Part model, mm, in its own coordinate system. A direction names the side the tool comes from. Coordinates: 2 decimals unless noted, no trailing zeros. Loops run counter-clockwise (first coordinate to the right, second up) from the corner with the lowest first, then second, coordinate; pieces in that order, holes last. Notation, with made-up numbers: M -19,-27.75 L 39,-27.75 A6 ccw 39,-17.75 Z; hole C 8.5,84.25 d5. An arc over 180 degrees is marked long. Use a Markdown table: item, result. Add a question column.
1) Tool access for faces 1 (the cylindrical face through (-1.46, 3.49, 6.59)), 2 (the flat face through (-2, 3, -6)): list every direction of +Z, -Z, +X, -X, +Y, -Y with a clear straight run to the whole face (end or side of a thin tool).
2) Pull direction Z, two halves, no side cores. Call faces 3 (the cylindrical face through (0, 2, 2)), 4 (the flat face through (-1, 4, -2)), 5 (the cylindrical face through (-6, 2, 0)): released by +Z, released by -Z, zero draft, split by the parting line, or undercut.
3) Band-saw the part on A-A (z = 0). List the corners of the cut face in (x, y).
4) Band-saw the part on C-C (y = 1.7). List the corners of the cut face in (x, z), plus the area to 3 significant figures.
5) Wall check: probe 1 along Z at (x, y) = (0, 1.35); probe 2 along Y at (x, z) = (-0.75, 6). Give the ranges that are in metal, low to high. Write a range as from..to.
6) Band-saw the part on B-B (x = 0). List the corners of the cut face in (y, z), plus the area to 3 significant figures.
7) Pin check, flat tips, straight feed: pin 1 Ø2 at (x, y) = (4, 2.5) entering from -Z; pin 2 Ø2 at (y, z) = (1.5, -5) entering from -X. Stop position of each tip, or through.
from build123d import *

# Parameters (mm, degrees)
CHAMFER_1_SIZE = 0.1


with BuildPart() as part:
    # 草图1 → 旋转1 (revolve)
    with BuildSketch(Plane.XY):
        Polygon((2, 0), (2, 4), (6.75, 4), (6.75, 3), (6, 3), (6, 0), align=None)
    revolve(axis=Axis((0, 0, 0), (0, 1, 0)))

    # 倒角1
    chamfer_1_edges = [part.edges().sort_by_distance(p)[0] for p in [
        (-6, 0, 0),
        (-6.75, 3, 0),
        (-6.75, 4, 0),
    ]]
    chamfer(chamfer_1_edges, length=CHAMFER_1_SIZE)


solid = part.part
Entries:
| question | item | result |
|---|---|---|
| 1 | face 1 | +Y, -Y |
| 1 | face 2 | -Y |
| 2 | face 3 | undercut |
| 2 | face 4 | zero draft |
| 2 | face 5 | split by the parting line |
| 3 | outline | M -6.75,3.1 L -6.65,3 L -6,3 L -6,0.1 L -5.9,0 L -2,0 L -2,4 L -6.65,4 L -6.75,3.9 Z; M 2,0 L 5.9,0 L 6,0.1 L 6,3 L 6.65,3 L 6.75,3.1 L 6.75,3.9 L 6.65,4 L 2,4 Z |
| 4 | outline | C 0,0 d12; hole C 0,0 d4 |
| 4 | area | 101 mm2 |
| 5 | probe 1 | -6..-2, 2..6 |
| 5 | probe 2 | 3..4 |
| 6 | outline | M 0,-5.9 L 0.1,-6 L 3,-6 L 3,-6.65 L 3.1,-6.75 L 3.9,-6.75 L 4,-6.65 L 4,-2 L 0,-2 Z; M 0,2 L 4,2 L 4,6.65 L 3.9,6.75 L 3.1,6.75 L 3,6.65 L 3,6 L 0.1,6 L 0,5.9 Z |
| 6 | area | 33.5 mm2 |
| 7 | pin 1 | z = -5.94 |
| 7 | pin 2 | x = -4.47 |
